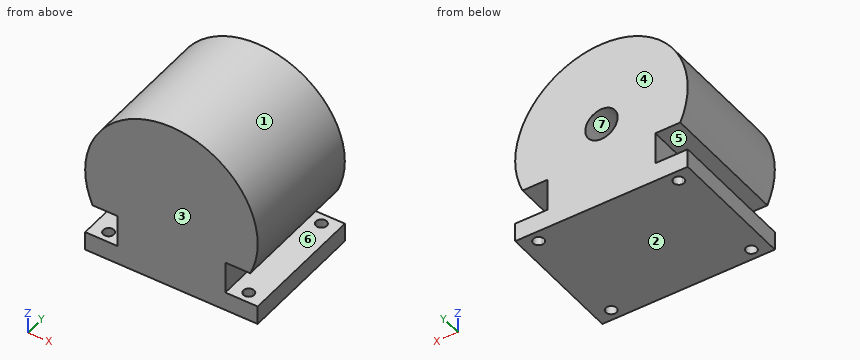
```python
from build123d import *

# Parameters (mm, degrees)
F0_W     = 15
F0_H     = 17.55002
F0_R     = 15
F2_DEPTH = 60
F3_DEPTH = 25
F4_DEPTH = 60


with BuildPart() as f2:
    # F0 (on Front) → F2 (new body, symmetric)
    with BuildSketch(Plane.XZ):
        with Locations((-72.5, 8.77501)):
            Rectangle(F0_W, F0_H)
        with BuildLine():
            Line((-65, 0), (0, 0))
            ThreePointArc((0, 0), (-26.495298, 4.514907), (-50, 17.55002))
            Line((-50, 17.55002), (-65, 17.55002))
            Line((-65, 17.55002), (-65, 0))
        make_face()
        with BuildLine():
            ThreePointArc((-50, 17.55002), (-26.495298, 4.514907), (0, 0))
            ThreePointArc((0, 0), (26.495298, 4.514907), (50, 17.55002))
            Line((50, 17.55002), (50, 47.55002))
            Line((50, 47.55002), (73.123176, 47.55002))
            ThreePointArc((73.123176, 47.55002), (0, 160), (-73.123176, 47.55002))
            Line((-73.123176, 47.55002), (-50, 47.55002))
            Line((-50, 47.55002), (-50, 17.55002))
        make_face()
        with Locations((0, 80)):
            Circle(F0_R, mode=Mode.SUBTRACT)
        with BuildLine():
            ThreePointArc((50, 17.55002), (26.495298, 4.514907), (0, 0))
            Line((0, 0), (65, 0))
            Line((65, 0), (65, 17.55002))
            Line((65, 17.55002), (50, 17.55002))
        make_face()
        with Locations((72.5, 8.77501)):
            Rectangle(F0_W, F0_H)
    extrude(amount=F2_DEPTH, both=True)

    # F1 (on Top) → F3 (cut)
    with BuildSketch(Plane.XY):
        with BuildLine():
            ThreePointArc((-60, 50), (-68.535534, 53.535534), (-65, 45))
            Line((-65, 45), (-65, 50))
            Line((-65, 50), (-60, 50))
        make_face()
        with BuildLine():
            Line((-65, 50), (-65, 45))
            ThreePointArc((-65, 45), (-61.464466, 46.464466), (-60, 50))
            Line((-60, 50), (-65, 50))
        make_face()
        with BuildLine():
            Line((-65, -45), (-65, -50))
            Line((-65, -50), (-60, -50))
            ThreePointArc((-60, -50), (-61.464466, -46.464466), (-65, -45))
        make_face()
        with BuildLine():
            Line((-60, -50), (-65, -50))
            Line((-65, -50), (-65, -45))
            ThreePointArc((-65, -45), (-68.535534, -53.535534), (-60, -50))
        make_face()
        with BuildLine():
            ThreePointArc((60, 50), (61.464466, 46.464466), (65, 45))
            Line((65, 45), (65, 50))
            Line((65, 50), (60, 50))
        make_face()
        with BuildLine():
            Line((65, 50), (65, 45))
            ThreePointArc((65, 45), (68.535534, 46.464466), (70, 50))
            ThreePointArc((70, 50), (65, 55), (60, 50))
            Line((60, 50), (65, 50))
        make_face()
        with BuildLine():
            Line((65, -50), (60, -50))
            ThreePointArc((60, -50), (65, -55), (70, -50))
            ThreePointArc((70, -50), (68.535534, -46.464466), (65, -45))
            Line((65, -45), (65, -50))
        make_face()
        with BuildLine():
            ThreePointArc((65, -45), (61.464466, -46.464466), (60, -50))
            Line((60, -50), (65, -50))
            Line((65, -50), (65, -45))
        make_face()
    extrude(amount=F3_DEPTH, mode=Mode.SUBTRACT)

    # F0 (on Front) → F4 (join, through all)
    with BuildSketch(Plane.XZ):
        with Locations((0, 80)):
            Circle(F0_R)
    extrude(amount=F4_DEPTH)


solid = f2.part
```
Build history of the part. All positions in model axes, mm. Face numbers are marked on the shaded views. A direction names the side the tool comes from. Round coordinates to 2 decimals unless told otherwise and drop trailing zeros. Loops run counter-clockwise (first coordinate to the right, second up) from the corner with the lowest first, then second, coordinate; pieces in that order, holes last.
Item 1: Which spindle directions (+Z, -Z, +X, -X, +Y, -Y) get a long thin tool onto all of the face, cutting with end or side? Do the marked faces 4, 5, 6 and 7. Say none if no direction does.
Item 2: Saw through at A-A (y = 3). List the corners of the cut face in (x, z), then the cut area to 3 significant figures.
Item 3: Saw through at B-B (x = 0). List the corners of the cut face in (y, z).
Item 4: Saw through at C-C (z = 80). List the corners of the cut face in (x, y).
Item 5: Pin check, flat tips, straight feed: P1, Ø11.5, axis at x = -65, y = -50, coming from the +Z side; P2, Ø2, axis at y = -14.5, z = 77, coming from the +X side (3 decimals); P3, Ø9, axis at x = -66.5, y = 7.5, coming from the +Z side. Stop position of each tip, or through.
Item 6: Saw through at D-D (y = -27). List the corners of the cut face in (x, z).
Item 7: Two-plate mould, pull along Z, no slides. Class the marked faces 1, 2 and 3: released by +Z, released by -Z, zero draft, split by the parting line, or undercut.
Item 8: Drill centre lines: line 1 along Y through (x, z) = (-65, 10.5); line 2 along X through (y, z) = (50, 9.5); line 3 along X through (y, z) = (1.5, 80.5). Where is each one in solid material? Low to high.
Worked answers:
1. face 4: +Z, -Z, +X, -X, +Y
1. face 5: -X, +Y, -Y
1. face 6: +X, +Y, -Y
1. face 7: +Y
2. outline: (-80, 0) - (80, 0) - (80, 17.55) - (50, 17.55) - (50, 47.55) - (73.12, 47.55) arc R80 ccw (long way) to (-73.12, 47.55) - (-50, 47.55) - (-50, 17.55) - (-80, 17.55) - close; hole circle Ø30 at (0, 80)
2. area: 20,200 mm2
3. outline: (-60, 0) - (60, 0) - (60, 65) - (0, 65) - (0, 95) - (60, 95) - (60, 160) - (-60, 160) - close
4. outline: (-80, -60) - (80, -60) - (80, 60) - (15, 60) - (15, 0) - (-15, 0) - (-15, 60) - (-80, 60) - close
5. P1: stops at z = 133.75
5. P2: stops at x = 79.975
5. P3: stops at z = 130.56
6. outline: (-80, 0) - (80, 0) - (80, 17.55) - (50, 17.55) - (50, 47.55) - (73.12, 47.55) arc R80 ccw (long way) to (-73.12, 47.55) - (-50, 47.55) - (-50, 17.55) - (-80, 17.55) - close
7. face 1: undercut
7. face 2: released by -Z
7. face 3: zero draft
8. line 1: y = -60 to -55, -45 to 45, 55 to 60
8. line 2: x = -80 to -70, -60 to 60, 70 to 80
8. line 3: x = -80 to -14.99, 14.99 to 80
